from build123d import *

# Parameters (mm, degrees)
F0_W     = 30
F0_H     = 25
F1_DEPTH = 400
F2_R     = 2
F3_R     = 10
F4_DEPTH = 400


with BuildPart() as f1:
    # F0 (on Front) → F1 (new body)
    with BuildSketch(Plane.XZ):
        Rectangle(F0_W, F0_H)
        with BuildLine():
            Line((-15, -12.5), (-15, 12.5))
            ThreePointArc((-15, 12.5), (-19.432726, 8.983673), (-22.111648, 4))
            Line((-22.111648, 4), (-15.19524, 4))
            Line((-15.19524, 4), (-15.19524, -4))
            Line((-15.19524, -4), (-22.111648, -4))
            ThreePointArc((-22.111648, -4), (-19.432726, -8.983673), (-15, -12.5))
        make_face()
        with BuildLine():
            ThreePointArc((-15, -12.5), (0, -16.519238), (15, -12.5))
            Line((15, -12.5), (-15, -12.5))
        make_face()
        with BuildLine():
            ThreePointArc((22.111648, 4), (19.432726, 8.983673), (15, 12.5))
            Line((15, 12.5), (15, -12.5))
            ThreePointArc((15, -12.5), (19.432726, -8.983673), (22.111648, -4))
            Line((22.111648, -4), (15.19524, -4))
            Line((15.19524, -4), (15.19524, 4))
            Line((15.19524, 4), (22.111648, 4))
        make_face()
        with BuildLine():
            Line((-15, 12.5), (15, 12.5))
            ThreePointArc((15, 12.5), (0, 16.082066), (-15, 12.5))
        make_face()
    extrude(amount=F1_DEPTH)

    # F2
    f2_edges = [f1.edges().sort_by_distance(p)[0] for p in [
        (-22.111648, -200, 4),
        (-15.19524, -200, 4),
        (-15.19524, -200, -4),
        (-22.111648, -200, -4),
        (15.19524, -200, -4),
        (22.111648, -200, 4),
        (15.19524, -200, 4),
        (22.111648, -200, -4),
    ]]
    fillet(f2_edges, radius=F2_R)

    # F3 (on face) → F4 (cut)
    with BuildSketch(Plane.XZ.offset(400)):
        Circle(F3_R)
    extrude(amount=-F4_DEPTH, mode=Mode.SUBTRACT)


solid = f1.part
Part model, mm, in its own coordinate system. Give positions to 0.01 mm unless a question says otherwise; leave off trailing zeros. Loops run counter-clockwise (first coordinate to the right, second up) from the corner with the lowest first, then second, coordinate; pieces in that order, holes last. Notation, with made-up numbers: M -34.5,-24 L -28.5,-24 A16 ccw -28.5,-6 Z; hole C -32.75,87 d10. An arc over 180 degrees is marked long. Put each result on its own line as item: value. Start each with the question number.
1) Pull direction Z, two halves, no side cores. Call faces 1 (the flat face through (-10, -400, -4)), 2 (the cylindrical face through (0.22, -197.2, 16.08)), 3 (the cylindrical face through (-2.17, -202.8, -9.76)): +Z half, -Z half, draft (parallel to the pull), parting line (faces both ways), or undercut.
2) Saw through at A-A (x = 0). List the corners of the cut face in (y, z).
3) Flat gauge pins, fed straight in: pin 1 (12 mm diameter, centred on x = -0.5, y = -278, fed in from +Z); pin 2 (0.9 mm diameter, centred on x = 18, y = -281, fed in from -Z); pin 3 (2 mm diameter, centred on y = -212.5, z = -0.5, fed in from -X); pin 4 (2 mm diameter, centred on x = -7, y = -228, fed in from -Z). Where does each tip first touch, or does it go through?
4) Saw through at B-B (y = -69). List the corners of the cut face in (x, z).
5) Probe probe 1 along X at (y, z) = (-228, -1); probe 2 along X at (y, z) = (-115, -8); probe 3 along Z at (x, y) = (-16, -242.5). List the from-to ranges inside material, lowest first.
Numbers:
1. face 1: draft
1. face 2: +Z half
1. face 3: undercut
2. outline: M -400,-16.52 L 0,-16.52 L 0,-10 L -400,-10 Z; M -400,10 L 0,10 L 0,16.08 L -400,16.08 Z
3. pin 1: z = 16.08
3. pin 2: z = -10.84
3. pin 3: x = -15.2
3. pin 4: z = -15.91
4. outline: M -20.82,-7 A14 ccw -15,-12.5 A30 ccw 15,-12.5 A14 ccw 20.82,-7 A2 ccw 19.09,-4 L 17.2,-4 A2 cw 15.2,-2 L 15.2,2 A2 cw 17.2,4 L 19.09,4 A2 ccw 20.82,7 A14 ccw 15,12.5 A33.2 ccw -15,12.5 A14 ccw -20.82,7 A2 ccw -19.09,4 L -17.2,4 A2 cw -15.2,2 L -15.2,-2 A2 cw -17.2,-4 L -19.09,-4 A2 ccw Z; hole C 0,0 d20
5. probe 1: -15.2 to -9.95, 9.95 to 15.2
5. probe 2: -20.18 to -6, 6 to 20.18
5. probe 3: -11.94 to -3.6, 3.6 to 11.94
